For this review, take the finished solid that the model builds, in its own axes (mm). A direction names the side the tool comes from. Coordinates: 2 decimals unless noted, no trailing zeros. Loops run counter-clockwise (first coordinate to the right, second up) from the corner with the lowest first, then second, coordinate; pieces in that order, holes last. Notation, with made-up numbers: (25, 32) -> (34, 32) arc R12 ccw to (34, 41) -> close; hole circle Ø8 at (-17, -37.5). An arc over 180 degrees is marked (long way). One line per item, written item: value.
Autodesk Inventor part; units mm, degrees
ref_plane "YZ Plane" through (0, 0, 0) normal (1, 0, 0) x (0, 1, 0)
ref_plane "XZ Plane" through (0, 0, 0) normal (0, 1, 0) x (-1, 0, 0)
ref_plane "XY Plane" through (0, 0, 0) normal (0, 0, 1) x (1, 0, 0)
sketch "Sketch1" plane through (0, 0, 0) normal (0, 1, 0) x (-1, 0, 0)
  line L0 (0, 0) -> (0, -20)
  line L1 (42, 0) -> (0, 0)
  line L2 (42, -10) -> (42, 0)
  line L3 (12, -10) -> (42, -10)
  line L4 (12, -20) -> (12, -10)
  line L5 (0, -20) -> (12, -20)
extrude "Extrusion1" add sketch "Sketch1" along normal blind 1.27
sketch "Sketch2" plane through (0, 1.27, 0) normal (0, 1, 0) x (1, 0, 0)
  point P0 (-6, 15)
hole "Hole1" at (-6, 1.27, -15) direction (0, -1, 0) diameter 4 depth 1.27
properties part number "Y-axis Carriage Flag" material "ABS Plastic"
1. To check wall thickness, follow probe 1 along X at (y, z) = (0.55, -15); probe 2 along Z at (x, y) = (-6, 0.7); probe 3 along X at (y, z) = (1.1, -17.5). State the ranges of each line that lie inside material, in increasing order. Write a range as from..to.
Return value:
probe 1: x = -12..-8, -4..0
probe 2: z = -20..-17, -13..0
probe 3: x = -12..0
2. Take a section at C-C, the plane x = -4.5. Give the boundary of the cut face in (y, z).
Return value:
outline: (0, -20) -> (1.27, -20) -> (1.27, -16.32) -> (0, -16.32) -> close; (0, -13.68) -> (1.27, -13.68) -> (1.27, 0) -> (0, 0) -> close
3. The part is to be moulded in two halves that separate along X. For faces 3 (the flat face through (-6, 1, -20)), 4 (the cylindrical face through (-8, 1, -15)), 5 (the flat face through (0, 1, -10)), 6 (the flat face through (-12, 1, -15)), say which applies: pulls with the +X half, pulls with the -X half, needs draft (parallel to the pull), parting line crosses it, or undercut.
Return value:
face 3: needs draft
face 4: undercut
face 5: pulls with the +X half
face 6: pulls with the -X half
4. Take a section at A-A, the plane y = 0.55. Give the boundary of the cut face in (x, z).
Return value:
outline: (-42, -10) -> (-12, -10) -> (-12, -20) -> (0, -20) -> (0, 0) -> (-42, 0) -> close; hole circle Ø4 at (-6, -15)
5. For faces 1 (the flat face through (-16, 1.27, -8)), 2 (the flat face through (-27, 1, -10)), list the 3-axis set-ups (+Z, -Z, +X, -X, +Y, -Y) from which the entire face can be reached by the end or side of a thin tool; tool diameter is ignored.
Return value:
face 1: +Z, -Z, +X, -X, +Y
face 2: -Z, -X, +Y, -Y
6. Insertion check: pin 1 Ø3 at (x, z) = (-6, -15) entering from +Y; pin 2 Ø0.6 at (x, y) = (-21.5, 0.5) entering from -Z. Each pin has a flat end and moves straight along its axis. Give the tip position at first contact, or say it passes through.
Return value:
pin 1: passes through
pin 2: stops at z = -10
7. Take a section at B-B, the plane z = -15. Give the boundary of the cut face in (x, y).
Return value:
outline: (-12, 0) -> (-8, 0) -> (-8, 1.27) -> (-12, 1.27) -> close; (-4, 0) -> (0, 0) -> (0, 1.27) -> (-4, 1.27) -> close
8. Take a section at D-D, the plane x = -17.5. Give the boundary of the cut face in (y, z).
Return value:
outline: (0, -10) -> (1.27, -10) -> (1.27, 0) -> (0, 0) -> close
